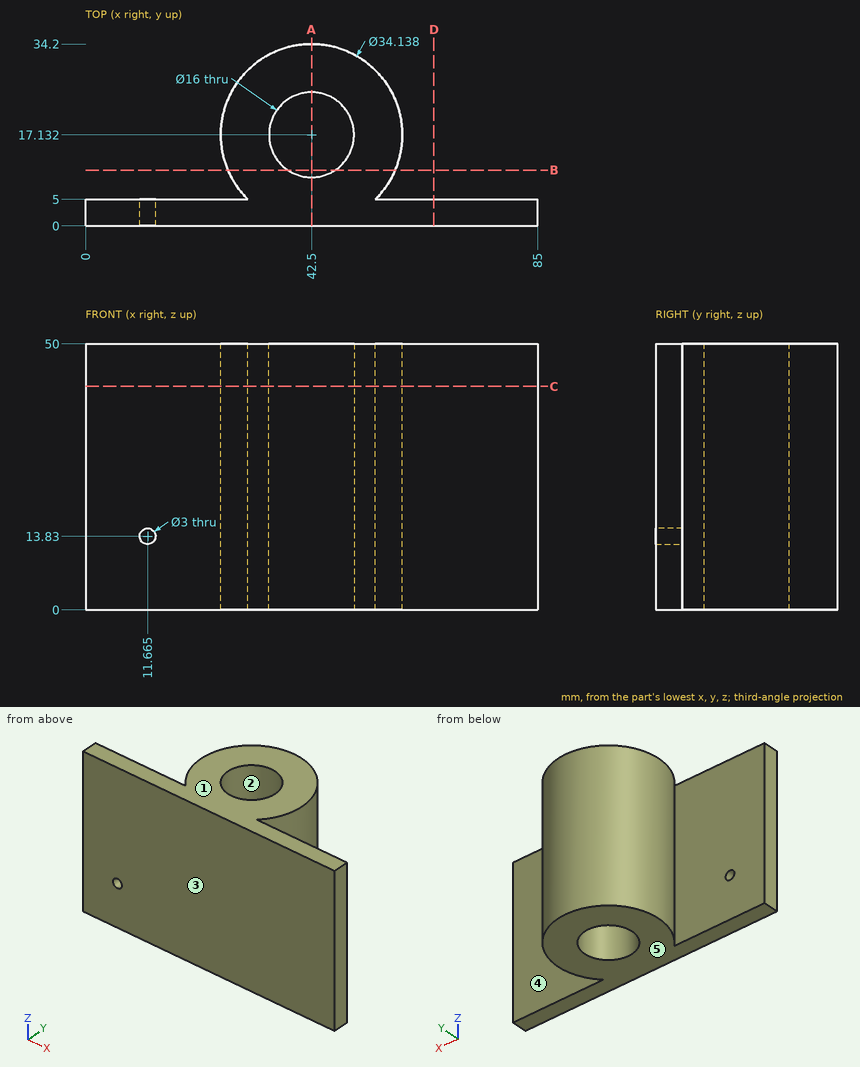
Study the drawing (mm; zero at the part's minimum x, y, z) and answer. A direction names the side the tool comes from. Give positions to 0.01 mm unless a question says otherwise; leave off trailing zeros. Loops run counter-clockwise (first coordinate to the right, second up) from the corner with the lowest first, then second, coordinate; pieces in that order, holes last. Notation, with made-up numbers: (24.5, -23) - (78.5, -23) arc R22 ccw to (78.5, 1) - close; hole circle Ø3 at (67, -5). An arc over 180 degrees is marked (long way). Answer in a Markdown table with one row per item. Add a question column.
Q1. The part is cut by section D-D (x = 65.5). Determine the outline of the cut face in (y, z), and give its area (3 significant figures).
Q2. The part is cut by section B-B (y = 10.5). Determine the outline of the cut face in (x, z) (1 decimal), and give its area (3 significant figures).
Q3. The part is cut by section C-C (z = 42). Determine the outline of the cut face in (x, y), and give its area (3 significant figures).
Q4. Each of these flat-tipped pins is pushed along its axis until it touches: P1, Ø2, axis at x = 28, z = 26.5, coming from the +Y side (1 decimal); P2, Ø15, axis at x = 71, z = 36.5, coming from the +Y side; P3, Ø8, axis at y = 30, z = 18, coming from the +X side (1 decimal); P4, Ø1.8, axis at x = 11.67, z = 13.83, coming from the -Y side. Where does it stop, or does it pass through?
Q5. A tool of negligible diameter and unlimited length cuts with its end or side. For the marked faces 4 and 5, from which of +Z, -Z, +X, -X, +Y, -Y can it reach the whole face along a straight path? Write none if from no direction.
Q6. Consider line 1 along Y through (x, z) = (42, 30) (1 decimal); line 2 along Y through (x, z) = (10.5, 46); line 3 along X through (y, z) = (12, 16.5). Determine where each line is inside the solid, lowest interval first.
Q7. Determine the mould class of the marked faces 1, 2 and 3 for opening direction Y: released by +Y, released by -Y, zero draft, split by the parting line, or undercut.
Q8. The part is cut by section A-A (x = 42.5). Determine the outline of the cut face in (y, z).
Solution:
| question | item | result |
|---|---|---|
| 1 | outline | (0, 0) - (5, 0) - (5, 50) - (0, 50) - close |
| 1 | area | 250 mm² |
| 2 | outline | (26.8, 0) - (38, 0) - (38, 50) - (26.8, 50) - close; (47, 0) - (58.2, 0) - (58.2, 50) - (47, 50) - close |
| 2 | area | 1,130 mm² |
| 3 | outline | (0, 0) - (85, 0) - (85, 5) - (54.51, 5) arc R17.07 ccw (long way) to (30.49, 5) - (0, 5) - close; hole circle Ø16 at (42.5, 17.13) |
| 3 | area | 1,060 mm² |
| 4 | P1 | stops at y = 27.6 |
| 4 | P2 | stops at y = 5 |
| 4 | P3 | stops at x = 57.1 |
| 4 | P4 | passes through |
| 5 | face 4 | +Z, -Z, +X |
| 5 | face 5 | -Z, +X, -X, +Y, -Y |
| 6 | line 1 | y = 0 to 9.1, 25.1 to 34.2 |
| 6 | line 2 | y = 0 to 5 |
| 6 | line 3 | x = 26.22 to 36.36, 48.64 to 58.78 |
| 7 | face 1 | zero draft |
| 7 | face 2 | undercut |
| 7 | face 3 | released by -Y |
| 8 | outline | (0, 0) - (9.13, 0) - (9.13, 50) - (0, 50) - close; (25.13, 0) - (34.2, 0) - (34.2, 50) - (25.13, 50) - close |
